For this review, take the finished solid that the model builds, in its own axes (mm). A direction names the side the tool comes from. Coordinates: 2 decimals unless noted, no trailing zeros. Write each loop counter-clockwise with the first axis right and the second up, starting at its lowest first coordinate (ties: lowest second). Pieces come first, ordered by that corner, then holes. Notation, with made-up numbers: M -27.5,21 L 8.5,21 A22 ccw 8.5,32 Z; hole C -23,58 d3. An arc over 180 degrees is marked long. Return JSON: item names as keys, results as strings.
```python
from build123d import *

# Parameters (mm, degrees)
BOSS_EXTRUDE1_DEPTH = 3
CUT_EXTRUDE2_DEPTH  = 10
SKETCH7_R           = 1
CUT_EXTRUDE3_DEPTH  = 11.5


with BuildPart() as part:
    # Sketch1 → Boss-Extrude1 (new body)
    with BuildSketch(Plane(origin=(0, 0, 0), x_dir=(1, 0, 0), z_dir=(0, 1, 0))):
        Polygon((-32, -43.117707706), (-20.011895516, -50), (20.011895516, -50), (32, -43.117707706), (32, 43.117707706), (20.011895516, 50), (-20.011895516, 50), (-32, 43.117707706), align=None)
    extrude(amount=BOSS_EXTRUDE1_DEPTH)

    # Sketch5 → Cut-Extrude2 (cut)
    with BuildSketch(Plane(origin=(0, 3, 0), x_dir=(1, 0, 0), z_dir=(0, 1, 0))):
        with BuildLine():
            Line((-14.620176413, -2.5), (14.620176413, -2.5))
            ThreePointArc((14.620176413, -2.5), (16.352588027, -1.782411614), (17.070176413, -0.05))
            Line((17.070176413, -0.05), (17.070176413, 0.05))
            ThreePointArc((17.070176413, 0.05), (16.352588027, 1.782411614), (14.620176413, 2.5))
            Line((14.620176413, 2.5), (-14.620176413, 2.5))
            ThreePointArc((-14.620176413, 2.5), (-16.352588027, 1.782411614), (-17.070176413, 0.05))
            Line((-17.070176413, 0.05), (-17.070176413, -0.05))
            ThreePointArc((-17.070176413, -0.05), (-16.352588027, -1.782411614), (-14.620176413, -2.5))
        make_face()
        with BuildLine():
            Line((14.45, -38.5), (14.55, -38.5))
            ThreePointArc((14.55, -38.5), (16.282411614, -37.782411614), (17, -36.05))
            Line((17, -36.05), (17, -15.95))
            ThreePointArc((17, -15.95), (16.282411614, -14.217588386), (14.55, -13.5))
            Line((14.55, -13.5), (14.45, -13.5))
            ThreePointArc((14.45, -13.5), (12.717588386, -14.217588386), (12, -15.95))
            Line((12, -15.95), (12, -36.05))
            ThreePointArc((12, -36.05), (12.717588386, -37.782411614), (14.45, -38.5))
        make_face()
        with BuildLine():
            Line((14.45, 13.5), (14.55, 13.5))
            ThreePointArc((14.55, 13.5), (16.282411614, 14.217588386), (17, 15.95))
            Line((17, 15.95), (17, 36.05))
            ThreePointArc((17, 36.05), (16.282411614, 37.782411614), (14.55, 38.5))
            Line((14.55, 38.5), (14.45, 38.5))
            ThreePointArc((14.45, 38.5), (12.717588386, 37.782411614), (12, 36.05))
            Line((12, 36.05), (12, 15.95))
            ThreePointArc((12, 15.95), (12.717588386, 14.217588386), (14.45, 13.5))
        make_face()
    extrude(amount=-CUT_EXTRUDE2_DEPTH, mode=Mode.SUBTRACT)

    # Sketch7 → Cut-Extrude3 (cut)
    with BuildSketch(Plane(origin=(0, 3, 0), x_dir=(1, 0, 0), z_dir=(0, 1, 0))):
        with Locations((-3, 28.2)):
            Circle(SKETCH7_R)
        with Locations((-3, 20.7)):
            Circle(SKETCH7_R)
        with Locations((-17, 20.7)):
            Circle(SKETCH7_R)
        with Locations((-17, 28.2)):
            Circle(SKETCH7_R)
    cut_extrude3 = extrude(amount=-CUT_EXTRUDE3_DEPTH, mode=Mode.SUBTRACT)

    # Mirror1: Cut-Extrude3 across plane
    add(cut_extrude3.mirror(Plane(origin=(0, 0, 0), x_dir=(1, 0, 0), z_dir=(0, 0, -1))), mode=Mode.SUBTRACT)


solid = part.part
```
1. We need section B-B (x = -6.5). State the section outline as (y, z) points, plus the area to 3 significant figures.
Checks:
{"outline": "M 0,-50 L 3,-50 L 3,-2.5 L 0,-2.5 Z; M 0,2.5 L 3,2.5 L 3,50 L 0,50 Z", "area": "285 mm2"}
2. Wall thickness on L1, parallel to X at y = 2, z = 28.2; L2, parallel to Z at x = -3, y = 2.2; L3, parallel to Z at x = 0, y = 2.85: over which ranges is each line inside the solid? List them lowest first. Write a range as from..to.
Checks:
{"L1": "-32..-18, -16..-4, -2..12, 17..32", "L2": "-50..-29.2, -27.2..-21.7, -19.7..-2.5, 2.5..19.7, 21.7..27.2, 29.2..50", "L3": "-50..-2.5, 2.5..50"}
3. For faces 5 (the face through (0, 2, -2.5)), 6 (the face through (-25.92, 1.48, -46.61)), list the 3-axis set-ups (+Z, -Z, +X, -X, +Y, -Y) from which the entire face can be reached by the end or side of a thin tool; tool diameter is ignored.
Checks:
{"face 5": "+Y, -Y", "face 6": "-Z, -X, +Y, -Y"}
4. Draft analysis for pull direction X (two halves, no side actions). For faces 1 (the face through (32, 1, 1)), 2 (the face through (-2.54, 1.52, -19.81)), 3 (the face through (0, 1, -50)), 4 (the face through (-3.217, 1.521, 27.224)), state which applies: +X half, -X half, draft (parallel to the pull), parting line (faces both ways), or undercut.
Checks:
{"face 1": "+X half", "face 2": "undercut", "face 3": "draft", "face 4": "undercut"}
5. We need section C-C (y = 1.45). Give the number of separate pieces and of enclosed holes in the cut face, plus the area to 3 significant figures.
Checks:
{"separate pieces": "1", "enclosed holes": "11", "area": "5,800 mm2"}
6. We need section D-D (x = -27.5). State the section outline as (y, z) points.
Checks:
{"outline": "M 0,-45.7 L 3,-45.7 L 3,45.7 L 0,45.7 Z"}
7. We need section A-A (z = 20.7). State the section outline as (x, y) points, plus the area to 3 significant figures.
Checks:
{"outline": "M -32,0 L -18,0 L -18,3 L -32,3 Z; M -16,0 L -4,0 L -4,3 L -16,3 Z; M -2,0 L 12,0 L 12,3 L -2,3 Z; M 17,0 L 32,0 L 32,3 L 17,3 Z", "area": "165 mm2"}
